from build123d import *

# Parameters (mm, degrees)
F0_W     = 807.72
F0_H     = 401.32
F1_DEPTH = 243.84
F2_R     = 60.96
F3_DEPTH = 45.72
F4_W     = 746.76
F4_H     = 340.36
F4_R     = 82.55
F4_R_2   = 60.96
F5_DEPTH = 45.72


with BuildPart() as f1:
    # F0 (on Top) → F1 (new body)
    with BuildSketch(Plane.XY):
        with Locations((12.259597, -118.231484)):
            Rectangle(F0_W, F0_H)
    extrude(amount=F1_DEPTH)

    # F2 (on face) → F3 (join)
    with BuildSketch(Plane.XY.offset(243.84)):
        with Locations((113.838267, -16.641684)):
            Circle(F2_R)
        with Locations((317.011298, -19.952157)):
            Circle(F2_R)
        with Locations((-298.568574, -219.742048)):
            Circle(F2_R)
        with Locations((-94.249569, -216.897499)):
            Circle(F2_R)
        with Locations((117.443508, -219.809698)):
            Circle(F2_R)
        with Locations((320.064545, -215.882391)):
            Circle(F2_R)
        with Locations((-89.340403, -13.697499)):
            Circle(F2_R)
        with Locations((-292.540403, -16.631484)):
            Circle(F2_R)
    extrude(amount=F3_DEPTH)

    # F4 (on Top) → F5 (join)
    with BuildSketch(Plane.XY):
        with Locations((12.259597, -118.231484)):
            Rectangle(F4_W, F4_H)
        with Locations((-208.453938, -102.044091)):
            Circle(F4_R, mode=Mode.SUBTRACT)
        with Locations((27.986567, -95.26559)):
            Circle(F4_R, mode=Mode.SUBTRACT)
        with Locations((240.385324, -99.75633)):
            Circle(F4_R, mode=Mode.SUBTRACT)
        with Locations((-208.453938, -102.044091)):
            Circle(F4_R_2)
        with Locations((27.986567, -95.26559)):
            Circle(F4_R_2)
        with Locations((240.385324, -99.75633)):
            Circle(F4_R_2)
    extrude(amount=F5_DEPTH)


solid = f1.part
For this review, take the finished solid that the model builds, in its own axes (mm). A direction names the side the tool comes from. Coordinates: 2 decimals unless noted, no trailing zeros. Loops run counter-clockwise (first coordinate to the right, second up) from the corner with the lowest first, then second, coordinate; pieces in that order, holes last. Notation, with made-up numbers: (26, 87) -> (30, 87) arc R27 ccw to (30, 123) -> close; hole circle Ø2 at (-24.5, -23). An arc over 180 degrees is marked (long way). Write each question's results on one line, items separated by ' | '.
Q1. Add section A-A, the plane z = 257. State the section outline as (x, y) points, then the cut area to 3 significant figures.
Taken from the geometry:
outline: circle Ø121.92 at (-298.57, -219.74); circle Ø121.92 at (-292.54, -16.63); circle Ø121.92 at (-94.25, -216.9); circle Ø121.92 at (-89.34, -13.7); circle Ø121.92 at (113.84, -16.64); circle Ø121.92 at (117.44, -219.81); circle Ø121.92 at (317.01, -19.95); circle Ø121.92 at (320.06, -215.88) | area: 93,400 mm²
Q2. For pin 1 Ø10 at (x, y) = (129.5, -120.5) entering from +Z, flat-tipped, find the tip position at first contact; note if it passes through.
Taken from the geometry:
pin 1: z = 243.84
Q3. Add section B-B, the plane x = 317. State the section outline as (y, z) points, then the cut area to 3 significant figures.
Taken from the geometry:
outline: (-318.89, 0) -> (82.43, 0) -> (82.43, 243.84) -> (41.01, 243.84) -> (41.01, 289.56) -> (-80.91, 289.56) -> (-80.91, 243.84) -> (-155, 243.84) -> (-155, 289.56) -> (-276.77, 289.56) -> (-276.77, 243.84) -> (-318.89, 243.84) -> close | area: 109,000 mm²
Q4. Machinability: for faces 1 (the flat face through (-90, -13, 289.56)), 2 (the cylindrical face through (256.11, -17.27, 266.38)), which of the approach directions +Z, -Z, +X, -X, +Y, -Y give a long, thin tool a straight path to every point of the face, cutting with its end or side? Answer none if there is none.
Taken from the geometry:
face 1: +Z, +X, -X, +Y, -Y | face 2: +Z
Q5. To check wall thickness, follow line 1 along Z through (x, y) = (281, 49); line 2 along X through (y, z) = (-232.5, 247); line 3 along Y through (x, z) = (-136, 249). State the ranges of each line that lie inside material, in increasing order. Write a range as [from, to].
Taken from the geometry:
line 1: [0, 243.84] | line 2: [-358.18, -238.96], [-153.18, -35.32], [57.82, 177.07], [261.41, 378.72] | line 3: [-261.32, -172.48], [-52.93, 25.53]
Q6. Add section D-D, the plane x = -248. State the section outline as (y, z) points, then the cut area to 3 significant figures.
Taken from the geometry:
outline: (-318.89, 0) -> (82.43, 0) -> (82.43, 243.84) -> (24.99, 243.84) -> (24.99, 289.56) -> (-58.25, 289.56) -> (-58.25, 243.84) -> (-185.7, 243.84) -> (-185.7, 289.56) -> (-253.79, 289.56) -> (-253.79, 243.84) -> (-318.89, 243.84) -> close | area: 105,000 mm²
Q7. Mouldability with a two-part tool opening along X and no side actions: class faces 3 (the cylindrical face through (-234.4, 1.7, 266.4)), 4 (the flat face through (117, -219, 289.56)), 5 (the flat face through (-391.6, -121, 120)) as +X half, -X half, draft (parallel to the pull), parting line (faces both ways), or undercut.
Taken from the geometry:
face 3: undercut | face 4: draft | face 5: -X half
Q8. Add section C-C, the plane y = -3.5. State the section outline as (x, z) points, then the cut area to 3 significant figures.
Taken from the geometry:
outline: (-391.6, 0) -> (416.12, 0) -> (416.12, 243.84) -> (375.71, 243.84) -> (375.71, 289.56) -> (258.31, 289.56) -> (258.31, 243.84) -> (173.36, 243.84) -> (173.36, 289.56) -> (54.31, 289.56) -> (54.31, 243.84) -> (-29.24, 243.84) -> (-29.24, 289.56) -> (-149.44, 289.56) -> (-149.44, 243.84) -> (-233.01, 243.84) -> (-233.01, 289.56) -> (-352.07, 289.56) -> (-352.07, 243.84) -> (-391.6, 243.84) -> close | area: 219,000 mm²
